Geometry check sheet. Reference: the model listing, model coordinates, mm. Coordinates: 2 decimals unless noted, no trailing zeros. Loops run counter-clockwise (first coordinate to the right, second up) from the corner with the lowest first, then second, coordinate; pieces in that order, holes last. Notation, with made-up numbers: (65, 26) -> (81, 26) arc R14 cw to (81, 52) -> close; hole circle Ø4 at (43.5, 52). An arc over 180 degrees is marked (long way). Answer as a JSON object with one key per item and string values.
from build123d import *

# Parameters (mm, degrees)
SKETCH_1_W      = 31.8
SKETCH_1_H      = 20.3
EXTRUDE_1_DEPTH = 10.2
SKETCH_2_R      = 0.25
EXTRUDE_2_DEPTH = 3.8
FILLET_1_R      = 2


with BuildPart() as part:
    # Эскиз1 → Бобышка-Вытянуть1 (new body)
    with BuildSketch(Plane(origin=(0, 0, 0), x_dir=(1, 0, 0), z_dir=(0, 1, 0))):
        Rectangle(SKETCH_1_W, SKETCH_1_H)
    extrude(amount=EXTRUDE_1_DEPTH)

    # Эскиз2 → Бобышка-Вытянуть2 (add)
    with BuildSketch(Plane.XZ):
        with Locations(Location((11.3, 7.6, 0), (0, 0, 90))):
            Circle(SKETCH_2_R)
        with Locations(Location((-11.5, 7.6, 0), (0, 0, 90))):
            Circle(SKETCH_2_R)
        with Locations(Location((-9, 7.6, 0), (0, 0, 90))):
            Circle(SKETCH_2_R)
        with Locations(Location((-9, -7.6, 0), (0, 0, 90))):
            Circle(SKETCH_2_R)
        with Locations(Location((-11.5, -7.6, 0), (0, 0, 90))):
            Circle(SKETCH_2_R)
        with Locations(Location((11.3, -7.6, 0), (0, 0, 90))):
            Circle(SKETCH_2_R)
    extrude(amount=EXTRUDE_2_DEPTH)

    # Скругление1
    fillet_1_edges = [part.edges().sort_by_distance(p)[0] for p in [
        (-15.9, 10.2, 0),
        (0, 10.2, 10.15),
        (15.9, 10.2, 0),
        (0, 10.2, -10.15),
        (15.9, 5.1, 10.15),
        (-15.9, 5.1, 10.15),
        (-15.9, 5.1, -10.15),
        (15.9, 5.1, -10.15),
    ]]
    fillet(fillet_1_edges, radius=FILLET_1_R)


solid = part.part
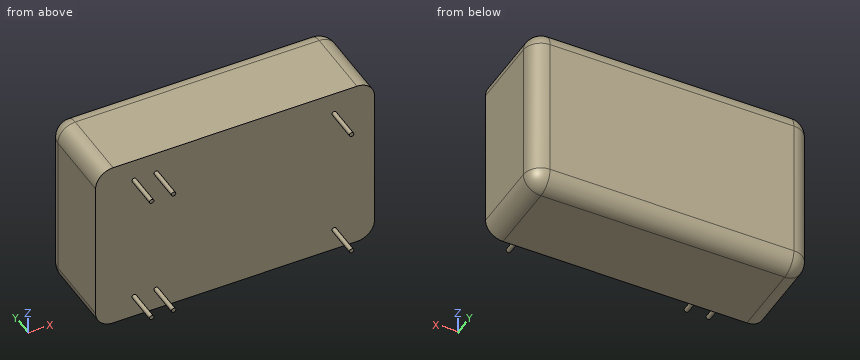
1. Section check A-A, the plane x = 13.5. Record the boundary of the cut face in (y, z), then the cut area to 3 significant figures.
Evaluation:
{"outline": "(0, -10.15) -> (8.2, -10.15) arc R2 ccw to (10.2, -8.15) -> (10.2, 8.15) arc R2 ccw to (8.2, 10.15) -> (0, 10.15) -> close", "area": "205 mm^2"}
2. Depth check by flat-ended pin: P1, Ø6, axis at x = 2, z = 4.5, coming from the -Y side. Enter the tip coordinate at first touch or a pass-through.
Evaluation:
{"P1": "stops at y = 0"}
3. Section check B-B, the plane z = 5. Record the boundary of the cut face in (x, y).
Evaluation:
{"outline": "(-15.9, 0) -> (15.9, 0) -> (15.9, 8.2) arc R2 ccw to (13.9, 10.2) -> (-13.9, 10.2) arc R2 ccw to (-15.9, 8.2) -> close"}
4. Thickness scan on probe 1 along Y at (x, z) = (4, -0.75); probe 2 along Z at (x, y) = (14, 5); probe 3 along X at (y, z) = (9, -2.25). Record the ranges inside material, lowest first. Write a range as from..to.
Evaluation:
{"probe 1": "y = 0..10.2", "probe 2": "z = -10.15..10.15", "probe 3": "x = -15.73..15.73"}
